```python
from build123d import *

# Parameters (mm, degrees)
SKETCH001_W             = 26.32
SKETCH001_H             = 32.67
PAD009_DEPTH            = 2
SKETCH004_R             = 3
SKETCH004_R_2           = 2
PAD010_DEPTH            = 3.3
SKETCH006_W             = 3.605088
SKETCH006_H             = 1.563431
PAD013_DEPTH            = 13
SKETCH015_R             = 2
POCKET_DEPTH            = 5.301
SKETCH016_W             = 13.978614
SKETCH016_H             = 3.56367
POCKET001_DEPTH         = 2.001
BODY002_PLACEMENT_ANGLE = 180


with BuildPart() as part:
    # Sketch001 → Pad009 (new body)
    with BuildSketch(Plane.XY):
        with Locations((12.7, 15.875)):
            Rectangle(SKETCH001_W, SKETCH001_H)
    extrude(amount=PAD009_DEPTH)

    # Sketch004 (on Face6 of Pad009) → Pad010 (join)
    with BuildSketch(Plane.XY.offset(2)):
        with Locations((2.54, 29.21)):
            Circle(SKETCH004_R)
        with Locations((2.54, 29.21)):
            Circle(SKETCH004_R_2, mode=Mode.SUBTRACT)
        with Locations((22.86, 29.21)):
            Circle(SKETCH004_R)
        with Locations((22.86, 29.21)):
            Circle(SKETCH004_R_2, mode=Mode.SUBTRACT)
        with Locations((22.86, 2.54)):
            Circle(SKETCH004_R)
        with Locations((22.86, 2.54)):
            Circle(SKETCH004_R_2, mode=Mode.SUBTRACT)
        with Locations((2.54, 2.54)):
            Circle(SKETCH004_R)
        with Locations((2.54, 2.54)):
            Circle(SKETCH004_R_2, mode=Mode.SUBTRACT)
    extrude(amount=PAD010_DEPTH)

    # Sketch006 (on Face1 of Pad010) → Pad013 (join)
    with BuildSketch(Plane(origin=(-0.46, 0, 0), x_dir=(0, -1, 0), z_dir=(-1, 0, 0))):
        with Locations((-30.41881, 0.781716)):
            Rectangle(SKETCH006_W, SKETCH006_H)
    extrude(amount=PAD013_DEPTH)

    # Sketch015 (on Face22 of Pad013) → Pocket (cut, through all)
    with BuildSketch(Plane.XY.offset(5.3)):
        with Locations((2.54, 29.21)):
            Circle(SKETCH015_R)
        with Locations((22.86, 29.21)):
            Circle(SKETCH015_R)
        with Locations((22.86, 2.54)):
            Circle(SKETCH015_R)
        with Locations((2.54, 2.54)):
            Circle(SKETCH015_R)
    extrude(amount=-POCKET_DEPTH, mode=Mode.SUBTRACT)

    # Sketch016 (on Face7 of Pocket) → Pocket001 (cut, through all)
    with BuildSketch(Plane.XY.offset(2)):
        with Locations((12.78762, 30.428165)):
            Rectangle(SKETCH016_W, SKETCH016_H)
    extrude(amount=-POCKET001_DEPTH, mode=Mode.SUBTRACT)


with BuildPart() as part_1:
    # Body002 placement: moved
    add(part.part.moved(Location((-9.46, 6, 68))).rotate(Axis((-9.46, 6, 68), (0, 0, 1)), BODY002_PLACEMENT_ANGLE))


solid = part_1.part
```
CAD build for the part. Positions are in the model's coordinates, mm. A direction names the side the tool comes from. Round coordinates to 2 decimals unless told otherwise and drop trailing zeros. Order: outer loops, then holes, each group sorted by start corner. A loop starts at its lowest first (then second) coordinate and runs counter-clockwise, first axis right, second up. Notation, with made-up numbers: (17.5, -19.5) - (49.5, -19.5) arc R15 ccw to (49.5, 4.5) - close; hole circle Ø10 at (37, 73.25). An arc over 180 degrees is marked (long way). Use CSV: the item, a comma, the result in double quotes. Start each with the question number.
1) Wall check: L1, parallel to Y at x = -12, z = 71.05; L2, parallel to Y at x = -32, z = 71.25; L3, parallel to Z at x = -27.5, y = -21. Give the ranges that are in metal, low to high. Write a range as [from, to].
2) Tool access for faces 4 (the cylindrical face through (-35.18, 2.56, 71.63)), 5 (the flat face through (-35, -26, 70)), 6 (the flat face through (-29.237, -24, 69)), 7 (the flat face through (-3, -22.616, 69)): list every direction of +Z, -Z, +X, -X, +Y, -Y with a clear straight run to the whole face (end or side of a thin tool).
3) Two-plate mould, pull along X, no slides. Class faces 1 (the cylindrical face through (-30.322, 3.372, 70.687)), 2 (the flat face through (-35, 6, 70)), 3 (the flat face through (-35.32, -10, 69)): pulls with the +X half, pulls with the -X half, needs draft (parallel to the pull), parting line crosses it, or undercut.
4) Saw through at C-C (y = -9.5). List the corners of the cut face in (x, z), and give its area (3 significant figures).
5) Saw through at B-B (x = -13.5). List the corners of the cut face in (y, z), and give its area (3 significant figures).
6) Saw through at D-D (x = -6). List the corners of the cut face in (y, z), and give its area (3 significant figures).
7) Saw through at A-A (z = 68.9). Count the separate pieces of the cut face and the enclosed holes in it, and give its area (3 significant figures).
8) Pin check, flat tips, straight feed: pin 1 Ø1.5 at (x, z) = (-1.5, 72) entering from -Y; pin 2 Ø0.6 at (x, z) = (-10.5, 69.5) entering from -Y; pin 3 Ø0.6 at (y, z) = (-7.5, 68.5) entering from +X; pin 4 Ø13 at (x, y) = (-25, -8.5) entering from +Z. Stop position of each tip, or through.
Values follow:
1,L1,"y = [-26.21, -25.21], [-21.21, -20.21], [0.46, 1.46], [5.46, 6.46]"
1,L2,"y = [-26.19, -25.18], [-21.24, -20.23], [0.48, 1.49], [5.43, 6.44]"
1,L3,"z = [68, 70]"
2,face 4,"+Z"
2,face 5,"+Z, -X, -Y"
2,face 6,"+Z, -Z, -Y"
2,face 7,"+Z, -Z, +X, +Y"
3,face 1,"undercut"
3,face 2,"needs draft"
3,face 3,"pulls with the -X half"
4,outline,"(-35.32, 68) - (-9, 68) - (-9, 70) - (-35.32, 70) - close"
4,area,"52.6 mm2"
5,outline,"(-26.21, 68) - (-24.53, 68) - (-24.53, 73.3) - (-25.81, 73.3) - (-25.81, 70) - (-26.21, 70) - close; (-21.89, 68) - (2.14, 68) - (2.14, 73.3) - (0.86, 73.3) - (0.86, 70) - (-20.61, 70) - (-20.61, 73.3) - (-21.89, 73.3) - close; (4.78, 68) - (6.46, 68) - (6.46, 70) - (6.06, 70) - (6.06, 73.3) - (4.78, 73.3) - close"
5,area,"71.6 mm2"
6,outline,"(-26.22, 68) - (-22.62, 68) - (-22.62, 69.56) - (-26.22, 69.56) - close"
6,area,"5.64 mm2"
7,separate pieces,"1"
7,enclosed holes,"4"
7,area,"807 mm2"
8,pin 1,"passes through"
8,pin 2,"stops at y = -26.21"
8,pin 3,"stops at x = -9"
8,pin 4,"stops at z = 70"
